Check sheet for the modelled part. Datum: model origin and axes. Units: mm. Face numbers are marked on the shaded views. Round coordinates to 2 decimals unless told otherwise and drop trailing zeros. Order: outer loops, then holes, each group sorted by start corner. A loop starts at its lowest first (then second) coordinate and runs counter-clockwise, first axis right, second up.
Q1. Scan lines: probe 1 along Y at (x, z) = (-14.5, 8.55); probe 2 along Y at (x, z) = (-5.5, 8.8); probe 3 along Y at (x, z) = (-7, 8.1). Record each from-to range of solid material in increasing order.
Q2. Mould release check, pull along Y, two halves, no side actions. Record for the marked faces 1 and 2: +Y half, -Y half, draft (parallel to the pull), parting line (faces both ways), or undercut.
Q3. Cross-section at C-C on x = 10.5. Record the cut outline in (y, z), then the cut area to 3 significant figures.
Q4. Depth check by flat-ended pin: P1, Ø1, axis at x = -4, y = 3, coming from the +Z side; P2, Ø1, axis at y = -6, z = 7, coming from the -X side; P3, Ø0.8, axis at y = -8, z = 7.5, coming from the +X side. Enter the tip coordinate at first touch or a pass-through.
Q5. Cross-section at B-B on y = -7.5. Record the cut outline in (x, z), then the cut area to 3 significant figures.
Q6. Cross-section at A-A on x = -10. Record the cut outline in (y, z), then the cut area to 3 significant figures.
Q7. Cross-section at D-D on y = 5.5. Record the cut outline in (x, z), then the cut area to 3 significant figures.
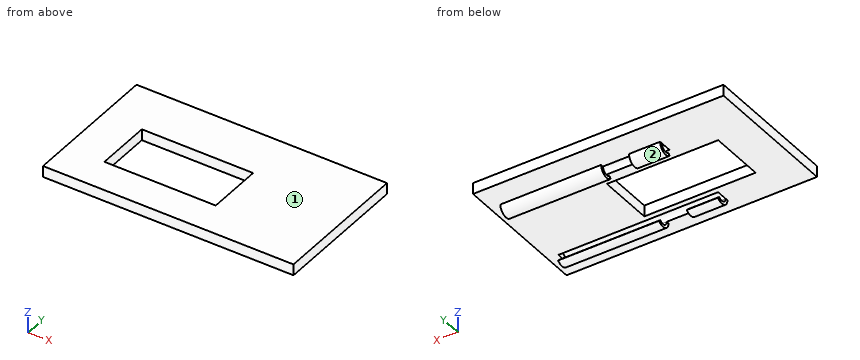
from build123d import *

# Parameters (mm, degrees)
Y_KSEKLIK_EKSTR_ZYON1_DEPTH = 10
BO_ALTMA1_T                 = -2
IZIM2_W                     = 45
IZIM2_H                     = 25
KES_EKSTR_ZYON1_DEPTH       = 8
IZIM3_W                     = 20
IZIM3_H                     = 10
KES_EKSTR_ZYON2_DEPTH       = 6
Y_KSEKLIK_EKSTR_ZYON2_DEPTH = 28.698952
KES_EKSTR_ZYON3_DEPTH       = 2.5


with BuildPart() as part:
    # Çizim1 → Yükseklik-Ekstrüzyon1 (new body)
    with BuildSketch(Plane.XY):
        Polygon((22.5, 11.5), (22.5, -11.5), (-22.5, -11.5), (-22.5, 11.5), (-22.5, 13.5), (22.5, 13.5), align=None)
    extrude(amount=Y_KSEKLIK_EKSTR_ZYON1_DEPTH)

    # İç Boşaltma1
    bo_altma1_openings = [part.faces().sort_by_distance(p)[0] for p in [
        (0, -11.5, 5),
        (-22.5, 1, 5),
        (22.5, 1, 5),
    ]]
    offset(amount=BO_ALTMA1_T, openings=bo_altma1_openings, kind=Kind.INTERSECTION)

    # Çizim2 → Kes-Ekstrüzyon1 (cut)
    with BuildSketch(Plane.XY):
        with Locations((0, 1)):
            Rectangle(IZIM2_W, IZIM2_H)
    extrude(amount=KES_EKSTR_ZYON1_DEPTH, mode=Mode.SUBTRACT)

    # Çizim3 → Kes-Ekstrüzyon2 (cut)
    with BuildSketch(Plane(origin=(0, 0, 8), x_dir=(-1, 0, 0), z_dir=(0, 0, -1))):
        with Locations((5.5, -0.5)):
            Rectangle(IZIM3_W, IZIM3_H)
    extrude(amount=-KES_EKSTR_ZYON2_DEPTH, mode=Mode.SUBTRACT)

    # Çizim4 → Kes-Döndür1 (revolve, cut)
    with BuildSketch(Plane(origin=(0, 0, 8), x_dir=(-1, 0, 0), z_dir=(0, 0, -1))):
        Polygon((-20.60881654, 7.5), (-20.60881654, 8.5), (-8.5, 8.5), (8.090135665, 8.5), (8.090135665, 7.5), align=None)
    kes_d_nd_r1 = revolve(axis=Axis((20.60881654, 7.5, 8), (-1, 0, 0)), mode=Mode.SUBTRACT)

    # Çizim6 → Yükseklik-Ekstrüzyon2 (add)
    with BuildSketch(Plane(origin=(-8.090135665, 0, 0), x_dir=(0, 0, -1), z_dir=(1, 0, 0))):
        with BuildLine():
            Line((-8, 9), (-8, 8.5))
            ThreePointArc((-8, 8.5), (-7.076120467, 7.882683432), (-7.292893219, 6.792893219))
            Line((-7.292893219, 6.792893219), (-6.939339828, 6.439339828))
            ThreePointArc((-6.939339828, 6.439339828), (-6.614180701, 8.074025149), (-8, 9))
        make_face()
    y_kseklik_ekstr_zyon2 = extrude(amount=Y_KSEKLIK_EKSTR_ZYON2_DEPTH)

    # Çizim8 → Kes-Ekstrüzyon3 (cut, symmetric)
    with BuildSketch(Plane(origin=(0, 0, 0), x_dir=(0, 0, -1), z_dir=(1, 0, 0))):
        with BuildLine():
            Line((-7.292893219, 6.792893219), (-6.939339828, 6.439339828))
            ThreePointArc((-6.939339828, 6.439339828), (-6.614180701, 8.074025149), (-8, 9))
            Line((-8, 9), (-8, 8.5))
            ThreePointArc((-8, 8.5), (-7.076120467, 7.882683432), (-7.292893219, 6.792893219))
        make_face()
    kes_ekstr_zyon3 = extrude(amount=KES_EKSTR_ZYON3_DEPTH, both=True, mode=Mode.SUBTRACT)

    # Aynalama1: Kes-Döndür1, Yükseklik-Ekstrüzyon2, Kes-Ekstrüzyon3 across plane
    add(kes_d_nd_r1.mirror(Plane.ZX), mode=Mode.SUBTRACT)
    add(y_kseklik_ekstr_zyon2.mirror(Plane.ZX))
    add(kes_ekstr_zyon3.mirror(Plane.ZX), mode=Mode.SUBTRACT)


solid = part.part
Results found:
1. probe 1: y = -11.5 to -5.5, 4.5 to 13.5
1. probe 2: y = -11.5 to -8.1, -6.9 to -5.5, 4.5 to 6.9, 8.1 to 13.5
1. probe 3: y = -11.5 to -8.49, -6.51 to -5.5, 4.5 to 6.51, 8.49 to 13.5
2. face 1: draft
2. face 2: undercut
3. outline: (-11.5, 8) - (-9, 8) arc R1.5 ccw to (-6.44, 6.94) - (-6.79, 7.29) arc R1 cw (long way) to (-6.5, 8) - (6.5, 8) arc R1 cw (long way) to (6.79, 7.29) - (6.44, 6.94) arc R1.5 ccw to (9, 8) - (13.5, 8) - (13.5, 10) - (-11.5, 10) - close
3. area: 49.8 mm2
4. P1: passes through
4. P2: stops at x = -8.09
4. P3: stops at x = 20.61
5. outline: (-22.5, 8) - (-8.09, 8) - (-8.09, 9) - (20.61, 9) - (20.61, 8) - (22.5, 8) - (22.5, 10) - (-22.5, 10) - close; (-8.09, 6.5) - (-2.5, 6.5) - (-2.5, 7) - (-8.09, 7) - close; (2.5, 6.5) - (20.61, 6.5) - (20.61, 7) - (2.5, 7) - close
5. area: 73.2 mm2
6. outline: (-11.5, 8) - (-5.5, 8) - (-5.5, 10) - (-11.5, 10) - close; (4.5, 8) - (13.5, 8) - (13.5, 10) - (4.5, 10) - close
6. area: 30.0 mm2
7. outline: (-22.5, 8) - (22.5, 8) - (22.5, 10) - (-22.5, 10) - close
7. area: 90.0 mm2
